For this review, take the finished solid that the model builds, in its own axes (mm). Give positions to 0.01 mm unless a question says otherwise; leave off trailing zeros.
Item 1: For P1, Ø6.5, axis at x = -1, z = 576, coming from the +Y side; P2, Ø1, axis at y = -17.5, z = 383, coming from the -X side; P3, Ø4, axis at x = 5, y = -4, coming from the -Z side; P4, Ø4, axis at y = 1, z = 517.5, coming from the +X side, all flat-tipped, find the tip position at first contact; note any pin that passes through.
Item 2: For probe 1 along X at (y, z) = (-5, 431.5); probe 2 along Y at (x, z) = (-14.5, 156), list the stretches that pass through material, from the lowest coordinate up.
Item 3: Consider section A-A (z = 737.5). Give the number of separate pieces and of enclosed holes in the cut face, plus the area to 3 significant figures.
```python
from build123d import *

# Parameters (mm, degrees)
BOSS_EXTRUDE1_DEPTH  = 810
MIRROR3_COPY_1_DEPTH = 810
MIRROR3_COPY_2_DEPTH = 810


with BuildPart() as part:
    # Sketch1 → Boss-Extrude1 (new body)
    with BuildSketch(Plane.XY):
        with BuildLine():
            Line((3.4, 0), (5.5, 0))
            Line((5.5, 0), (5.5, 4))
            Line((5.5, 4), (11.69, 10.19))
            Line((11.69, 10.19), (18.2, 10.19))
            Line((18.2, 10.19), (18.2, 5.265595036))
            Line((18.2, 5.265595036), (15.5, 5.265595036))
            Line((15.5, 5.265595036), (15.5, 2.965595036))
            Line((15.5, 2.965595036), (19, 2.965595036))
            Line((19, 2.965595036), (19, 3.965595036))
            Line((19, 3.965595036), (20, 3.965595036))
            Line((20, 3.965595036), (20, 15.5))
            ThreePointArc((20, 15.5), (18.681980515, 18.681980515), (15.5, 20))
            Line((15.5, 20), (6.385304712, 20))
            Line((6.385304712, 20), (6.385304712, 19))
            Line((6.385304712, 19), (5.385304712, 19))
            Line((5.385304712, 19), (5.385304712, 15.5))
            Line((5.385304712, 15.5), (7.685304712, 15.5))
            Line((7.685304712, 15.5), (7.685304712, 18.2))
            Line((7.685304712, 18.2), (10.19, 18.2))
            Line((10.19, 18.2), (10.19, 11.69))
            Line((10.19, 11.69), (4, 5.5))
            Line((4, 5.5), (0, 5.5))
            Line((0, 5.5), (0, 3.4))
            ThreePointArc((0, 3.4), (2.404163056, 2.404163056), (3.4, 0))
        make_face()
        with BuildLine():
            Line((18.5, 11.69), (18.5, 15.5))
            ThreePointArc((18.5, 15.5), (17.621320344, 17.621320344), (15.5, 18.5))
            Line((15.5, 18.5), (11.69, 18.5))
            Line((11.69, 18.5), (11.69, 11.69))
            Line((11.69, 11.69), (18.5, 11.69))
        make_face(mode=Mode.SUBTRACT)
    boss_extrude1 = extrude(amount=BOSS_EXTRUDE1_DEPTH)

    # Mirror1: Boss-Extrude1 across plane
    add(boss_extrude1.mirror(Plane.ZX))

    # Mirror2: Boss-Extrude1 across plane
    add(boss_extrude1.mirror(Plane(origin=(0, 0, 0), x_dir=(0, 0, 1), z_dir=(1, 0, 0))))

    # Mirror3 copy 1 sketch → Mirror3 copy 1 (add)
    with BuildSketch(Plane(origin=(0, 0, 0), x_dir=(-1, 0, 0), z_dir=(0, 0, 1))):
        with BuildLine():
            Line((3.4, 0), (5.5, 0))
            Line((5.5, 0), (5.5, 4))
            Line((5.5, 4), (11.69, 10.19))
            Line((11.69, 10.19), (18.2, 10.19))
            Line((18.2, 10.19), (18.2, 5.265595036))
            Line((18.2, 5.265595036), (15.5, 5.265595036))
            Line((15.5, 5.265595036), (15.5, 2.965595036))
            Line((15.5, 2.965595036), (19, 2.965595036))
            Line((19, 2.965595036), (19, 3.965595036))
            Line((19, 3.965595036), (20, 3.965595036))
            Line((20, 3.965595036), (20, 15.5))
            ThreePointArc((20, 15.5), (18.681980515, 18.681980515), (15.5, 20))
            Line((15.5, 20), (6.385304712, 20))
            Line((6.385304712, 20), (6.385304712, 19))
            Line((6.385304712, 19), (5.385304712, 19))
            Line((5.385304712, 19), (5.385304712, 15.5))
            Line((5.385304712, 15.5), (7.685304712, 15.5))
            Line((7.685304712, 15.5), (7.685304712, 18.2))
            Line((7.685304712, 18.2), (10.19, 18.2))
            Line((10.19, 18.2), (10.19, 11.69))
            Line((10.19, 11.69), (4, 5.5))
            Line((4, 5.5), (0, 5.5))
            Line((0, 5.5), (0, 3.4))
            ThreePointArc((0, 3.4), (2.404163056, 2.404163056), (3.4, 0))
        make_face()
        with BuildLine():
            Line((18.5, 11.69), (18.5, 15.5))
            ThreePointArc((18.5, 15.5), (17.621320344, 17.621320344), (15.5, 18.5))
            Line((15.5, 18.5), (11.69, 18.5))
            Line((11.69, 18.5), (11.69, 11.69))
            Line((11.69, 11.69), (18.5, 11.69))
        make_face(mode=Mode.SUBTRACT)
    extrude(amount=MIRROR3_COPY_1_DEPTH)

    # Mirror3 copy 2 sketch → Mirror3 copy 2 (add)
    with BuildSketch(Plane.XY):
        with BuildLine():
            Line((3.4, 0), (5.5, 0))
            Line((5.5, 0), (5.5, -4))
            Line((5.5, -4), (11.69, -10.19))
            Line((11.69, -10.19), (18.2, -10.19))
            Line((18.2, -10.19), (18.2, -5.265595036))
            Line((18.2, -5.265595036), (15.5, -5.265595036))
            Line((15.5, -5.265595036), (15.5, -2.965595036))
            Line((15.5, -2.965595036), (19, -2.965595036))
            Line((19, -2.965595036), (19, -3.965595036))
            Line((19, -3.965595036), (20, -3.965595036))
            Line((20, -3.965595036), (20, -15.5))
            ThreePointArc((20, -15.5), (18.681980515, -18.681980515), (15.5, -20))
            Line((15.5, -20), (6.385304712, -20))
            Line((6.385304712, -20), (6.385304712, -19))
            Line((6.385304712, -19), (5.385304712, -19))
            Line((5.385304712, -19), (5.385304712, -15.5))
            Line((5.385304712, -15.5), (7.685304712, -15.5))
            Line((7.685304712, -15.5), (7.685304712, -18.2))
            Line((7.685304712, -18.2), (10.19, -18.2))
            Line((10.19, -18.2), (10.19, -11.69))
            Line((10.19, -11.69), (4, -5.5))
            Line((4, -5.5), (0, -5.5))
            Line((0, -5.5), (0, -3.4))
            ThreePointArc((0, -3.4), (2.404163056, -2.404163056), (3.4, 0))
        make_face()
        with BuildLine():
            Line((18.5, -11.69), (18.5, -15.5))
            ThreePointArc((18.5, -15.5), (17.621320344, -17.621320344), (15.5, -18.5))
            Line((15.5, -18.5), (11.69, -18.5))
            Line((11.69, -18.5), (11.69, -11.69))
            Line((11.69, -11.69), (18.5, -11.69))
        make_face(mode=Mode.SUBTRACT)
    extrude(amount=MIRROR3_COPY_2_DEPTH)


solid = part.part
```
Resolved:
1. P1: stops at y = 5.75
1. P2: stops at x = -19.74
1. P3: stops at z = 0
1. P4: stops at x = 19
2. probe 1: x = -20 to -15.5, -6.5 to 6.5, 15.5 to 20
2. probe 2: y = -20 to -18.5, -11.69 to -10.19, 10.19 to 11.69, 18.5 to 20
3. separate pieces: 1
3. enclosed holes: 5
3. area: 468 mm2
